```python
from build123d import *

# Parameters (mm, degrees)
F0_R      = 1.5875
F1_DEPTH  = 12.7
F3_DEPTH  = 1.27
F5_DEPTH  = 1.27
F7_D      = 2.5273
F8_W      = 15.6464
F8_H      = 6.4008
F9_DEPTH  = 32.767
F11_DEPTH = 26.1494109194
F13_R     = 0.5969
F14_DEPTH = 4.2418


with BuildPart() as f1:
    # F0 (on Front) → F1 (new body)
    with BuildSketch(Plane.XZ):
        with BuildLine():
            Line((0, 12.7), (0, 0))
            Line((0, 0), (7.62, 0))
            Line((7.62, 0), (22.5517244204, 25.0878578359))
            ThreePointArc((22.5517244204, 25.0878578359), (21.0572314123, 31.8770293487), (14.1866754903, 30.817869066))
            Line((14.1866754903, 30.817869066), (0, 12.7))
        make_face()
        with Locations((18.1864, 27.686)):
            Circle(F0_R, mode=Mode.SUBTRACT)
    extrude(amount=F1_DEPTH)

    # F2 (on face) → F3 (cut)
    with BuildSketch(Plane.XZ.offset(12.7)):
        with BuildLine():
            ThreePointArc((5.2733546579, 2.54), (6.0579673524, 2.7474495771), (6.6375185393, 3.3155805737))
            Line((6.6375185393, 3.3155805737), (15.6851948134, 18.5172284021))
            ThreePointArc((15.6851948134, 18.5172284021), (15.8374637284, 19.7988156089), (14.9874738748, 20.7699844097))
            ThreePointArc((14.9874738748, 20.7699844097), (13.8801528815, 21.3994559769), (12.8931539876, 22.2045816934))
            ThreePointArc((12.8931539876, 22.2045816934), (11.6805013198, 22.6463113598), (10.5404804924, 22.0413286293))
            Line((10.5404804924, 22.0413286293), (2.8775860907, 12.2550106486))
            ThreePointArc((2.8775860907, 12.2550106486), (2.6267677486, 11.7939490899), (2.54, 11.2763015655))
            Line((2.54, 11.2763015655), (2.54, 4.1275))
            ThreePointArc((2.54, 4.1275), (3.0049679849, 3.0049679849), (4.1275, 2.54))
            Line((4.1275, 2.54), (5.2733546579, 2.54))
        make_face()
    extrude(amount=-F3_DEPTH, mode=Mode.SUBTRACT)

    # F4 (on face) → F5 (cut)
    with BuildSketch(Plane(origin=(0, 0, 0), x_dir=(-1, 0, 0), z_dir=(0, 1, 0))):
        with BuildLine():
            ThreePointArc((-2.54, 11.2763015655), (-2.6267677486, 11.7939490899), (-2.8775860907, 12.2550106486))
            Line((-2.8775860907, 12.2550106486), (-10.5404804924, 22.0413286293))
            ThreePointArc((-10.5404804924, 22.0413286293), (-11.6805013198, 22.6463113598), (-12.8931539876, 22.2045816934))
            ThreePointArc((-12.8931539876, 22.2045816934), (-13.8801528815, 21.3994559769), (-14.9874738748, 20.7699844097))
            ThreePointArc((-14.9874738748, 20.7699844097), (-15.8374637284, 19.7988156089), (-15.6851948134, 18.5172284021))
            Line((-15.6851948134, 18.5172284021), (-6.6375185393, 3.3155805737))
            ThreePointArc((-6.6375185393, 3.3155805737), (-6.0579673524, 2.7474495771), (-5.2733546579, 2.54))
            Line((-5.2733546579, 2.54), (-4.1275, 2.54))
            ThreePointArc((-4.1275, 2.54), (-3.0049679849, 3.0049679849), (-2.54, 4.1275))
            Line((-2.54, 4.1275), (-2.54, 11.2763015655))
        make_face()
    extrude(amount=-F5_DEPTH, mode=Mode.SUBTRACT)

    # F7 (through all)
    with Locations(Plane(origin=(0, 0, 0), x_dir=(0, -1, 0), z_dir=(-1, 0, 0))):
        with Locations((6.35, 2.54), (6.35, 10.16)):
            Hole(F7_D / 2)

    # F8 (on face) → F9 (cut, through all)
    with BuildSketch(Plane(origin=(0, 0, 0), x_dir=(1, 0, 0), z_dir=(0, 0, -1))):
        with Locations((15.4432, 6.2484)):
            Rectangle(F8_W, F8_H)
    extrude(amount=-F9_DEPTH, mode=Mode.SUBTRACT)

    # F10 (on face) → F11 (cut, through all)
    with BuildSketch(Plane(origin=(-6.1646719805, 0, 4.8270688221), x_dir=(0, -1, 0), z_dir=(-0.7873473444, 0, 0.6165096587))):
        with BuildLine():
            ThreePointArc((3.048, 22.3592149561), (6.2484, 19.1588149561), (9.4488, 22.3592149561))
            Line((9.4488, 22.3592149561), (3.048, 22.3592149561))
        make_face()
    extrude(amount=-F11_DEPTH, mode=Mode.SUBTRACT)

    # F13 (on offset) → F14 (cut)
    with BuildSketch(Plane.YZ.offset(23.4188)):
        with Locations((-11.0744, 27.686)):
            Circle(F13_R)
    extrude(amount=-F14_DEPTH, mode=Mode.SUBTRACT)


solid = f1.part
```
Could you check a few things on this model? Use its own coordinates, in mm. A direction names the side the tool comes from. Coordinates: 2 decimals unless noted, no trailing zeros. Write each loop counter-clockwise with the first axis right and the second up, starting at its lowest first coordinate (ties: lowest second). Pieces come first, ordered by that corner, then holes. Notation, with made-up numbers: (69, 48) -> (99, 48) arc R23 ccw to (99, 67) -> close; hole circle Ø11 at (72.5, 58). An arc over 180 degrees is marked (long way). Write item = value, one per line. Start each with the question number.
(1) I want a section at A-A (y = -6.25). Please give me the cut outline in (x, z).
(2) Which directions (+Z, -Z, +X, -X, +Y, -Y) give clear straight access to the entire face, cutting with the end or side of a thin tool? Please do faces 1 (the face through (5, -12, 2.54)), 2 (the face through (7.62, -6.2, 8.6)), 3 (the face through (3.863, -6.624, 8.926)), 4 (the face through (6.068, -0.626, 2.753)), 5 (the face through (6.401, -6.178, 19.322)).
(3) I need wall thicknesses on line 1 (Z direction, x = 3.25, y = -6.35); line 2 (Y direction, x = 11.5, z = 25); line 3 (Z direction, x = 4, y = -6.5). Which ranges of each line are inside material? Lowest first, please. Write a range as [from, to].
(4) I want a section at B-B (x = 19). Please give me the cut outline in (y, z), plus the area to 3 significant figures.
(5) I want a section at C-C (z = 10.16). Please give me the cut outline in (x, y), plus the area to 3 significant figures.
(6) We'd pull the mould along Z, two halves only. Please class faces 6 (the face through (15, 0, 16)), 7 (the face through (11.225, -0.626, 11.023)), 8 (the face through (5.616, -7.672, 19.873)), 9 (the face through (15, -11.1, 12.4)): released by +Z, released by -Z, zero draft, split by the parting line, or undercut.
(7) Will these pins go through, and if not, where does the flat tip stop? pin 1 (0.9 mm diameter, centred on x = 4.5, y = -1, fed in from +Z); pin 2 (1.1 mm diameter, centred on y = -11.07, z = 27.69, fed in from +X); pin 3 (5 mm diameter, centred on x = 11, z = 17, fed in from -Y).
(8) I want a section at D-D (z = 26.5). Please give me the cut outline in (x, y).
Result set:
q1.outline = (0, 0) -> (7.62, 0) -> (7.62, 1.28) -> (0, 1.28) -> close; (0, 3.8) -> (7.62, 3.8) -> (7.62, 8.9) -> (0, 8.9) -> close; (0, 11.42) -> (7.62, 11.42) -> (7.62, 18.37) -> (5.65, 19.91) -> (0, 12.7) -> close
q2.face_1 = -Y
q2.face_2 = +Z, -Z, +X
q2.face_3 = +X, -X
q2.face_4 = +Y
q2.face_5 = +Z, +X
q3.line_1 = [0, 1.28], [3.8, 8.9], [11.42, 16.85]
q3.line_2 = [-12.7, -9.45], [-3.05, 0]
q3.line_3 = [0, 1.29], [3.79, 8.91], [11.41, 17.81]
q4.outline = (-12.7, 19.12) -> (-9.45, 19.12) -> (-9.45, 26.32) -> (-12.7, 26.32) -> close; (-12.7, 29.05) -> (-9.45, 29.05) -> (-9.45, 32.7) -> (-12.7, 32.7) -> close; (-3.05, 19.12) -> (0, 19.12) -> (0, 26.32) -> (-3.05, 26.32) -> close; (-3.05, 29.05) -> (0, 29.05) -> (0, 32.7) -> (-3.05, 32.7) -> close
q4.area = 68.4 mm2
q5.outline = (0, -12.7) -> (2.54, -12.7) -> (2.54, -11.43) -> (10.71, -11.43) -> (10.71, -12.7) -> (13.67, -12.7) -> (13.67, -9.45) -> (7.62, -9.45) -> (7.62, -7.61) -> (0, -7.61) -> close; (0, -5.09) -> (7.62, -5.09) -> (7.62, -3.05) -> (13.67, -3.05) -> (13.67, 0) -> (10.71, 0) -> (10.71, -1.27) -> (2.54, -1.27) -> (2.54, 0) -> (0, 0) -> close
q5.area = 94.9 mm2
q6.face_6 = zero draft
q6.face_7 = undercut
q6.face_8 = released by +Z
q6.face_9 = released by -Z
q7.pin_1 = 19.02
q7.pin_2 = 16.7
q7.pin_3 = -11.43
q8.outline = (10.81, -12.7) -> (17.13, -12.7) -> (17.13, -9.45) -> (10.81, -9.45) -> close; (10.81, -3.05) -> (17.13, -3.05) -> (17.13, 0) -> (10.81, 0) -> close; (19.24, -12.7) -> (23.13, -12.7) -> (23.13, -9.45) -> (19.24, -9.45) -> close; (19.24, -3.05) -> (23.13, -3.05) -> (23.13, 0) -> (19.24, 0) -> close
